Design review of the part built by this model. Coordinates are the model's own, in mm. A direction names the side the tool comes from. Give positions to 0.01 mm unless a question says otherwise; leave off trailing zeros. Loops run counter-clockwise (first coordinate to the right, second up) from the corner with the lowest first, then second, coordinate; pieces in that order, holes last. Notation, with made-up numbers: (-26.5, -32) -> (-6.5, -32) arc R32 ccw to (-6.5, -6) -> close; hole circle Ø5 at (47.5, 77.25). An arc over 180 degrees is marked (long way). Use a Markdown table: item, result. Add a question column.
1. Add section A-A (y = 0). State the section outline as (x, z) points, and give its area (3 significant figures).
2. Add section B-B (z = 22). State the section outline as (x, y) points, and give its area (3 significant figures).
3. Draft analysis for pull direction Y (two halves, no side actions). For faces 1 (the flat face through (-43, 16, 26)), 2 (the flat face through (0, -30, 20)), 3 (the flat face through (9, -35, 3)), 4 (the flat face through (-2, 33, 23)), state which applies: pulls with the +Y half, pulls with the -Y half, needs draft (parallel to the pull), parting line crosses it, or undercut.
4. For faces 5 (the flat face through (-43, 16, 13)), 6 (the flat face through (42, 0, 23)), 7 (the flat face through (-2, 7, 40)), 8 (the flat face through (3.5, 0, 42)), list the 3-axis set-ups (+Z, -Z, +X, -X, +Y, -Y) from which the entire face can be reached by the end or side of a thin tool; tool diameter is ignored.
5. Add section C-C (x = 0). State the section outline as (y, z) points.
6. To check wall thickness, follow line 1 (Y direction, x = 0, z = 0.75); line 2 (X direction, y = -6, z = 34.5); line 3 (Y direction, x = 12.5, z = 11.5). State the ranges of each line that lie inside material, in increasing order.
7. For pin 1 Ø1 at (y, z) = (4.5, 15.5) entering from +X; pin 2 Ø12 at (y, z) = (15, 28.5) entering from -X; pin 3 Ø8 at (x, y) = (0, 40) entering from -Z; pin 4 Ø6 at (y, z) = (-22, 5.5) entering from -X, all flat-tipped, find the tip position at first contact; note any pin that passes through.
8. Add section D-D (z = 35). State the section outline as (x, y) points.
```python
from build123d import *

# Parameters (mm, degrees)
F0_R     = 60
F0_R_2   = 5
F0_W     = 86
F0_H     = 66
F1_DEPTH = 3
F2_DEPTH = 40
F3_W     = 86
F3_H     = 66
F4_DEPTH = 3
F5_W     = 10
F5_H     = 12
F5_W_2   = 13
F5_H_2   = 13
F6_DEPTH = 25
F8_DEPTH = 25


with BuildPart() as f1:
    # F0 (on Top) → F1 (new body)
    with BuildSketch(Plane.XY):
        Circle(F0_R)
        with Locations((0, -40)):
            Circle(F0_R_2, mode=Mode.SUBTRACT)
        with Locations((-1, 0)):
            Rectangle(F0_W, F0_H, mode=Mode.SUBTRACT)
        with Locations((0, 40)):
            Circle(F0_R_2, mode=Mode.SUBTRACT)
    extrude(amount=F1_DEPTH)

    # F0 (on Top) → F2 (join)
    with BuildSketch(Plane.XY):
        with Locations((-1, 0)):
            Rectangle(F0_W, F0_H)
        Polygon((39, 30), (39, 2), (39, -30), (-41, -30), (-41, 0), (-41, 30), align=None, mode=Mode.SUBTRACT)
    extrude(amount=F2_DEPTH)

    # F3 (on face) → F4 (join)
    with BuildSketch(Plane.XY.offset(40)):
        with Locations((-1, 0)):
            Rectangle(F3_W, F3_H)
    extrude(amount=F4_DEPTH)

    # F5 (on face) → F6 (cut)
    with BuildSketch(Plane(origin=(-44, 0, 0), x_dir=(0, -1, 0), z_dir=(-1, 0, 0))):
        with Locations((14.5, 19)):
            Rectangle(F5_W, F5_H)
        with Locations((-15.9, 19.5)):
            Rectangle(F5_W_2, F5_H_2)
    extrude(amount=-F6_DEPTH, mode=Mode.SUBTRACT)

    # F7 (on face) → F8 (cut)
    with BuildSketch(Plane.XY.offset(43)):
        Polygon((3.5, -3.1), (3.5, 0), (3.5, 3.1), (-3.5, 3.1), (-3.5, 0), (-3.5, -3.1), align=None)
    extrude(amount=-F8_DEPTH, mode=Mode.SUBTRACT)


solid = f1.part
```
Taken from the geometry:
| question | item | result |
|---|---|---|
| 1 | outline | (-60, 0) -> (-41, 0) -> (-41, 40) -> (-3.5, 40) -> (-3.5, 43) -> (-44, 43) -> (-44, 3) -> (-60, 3) -> close; (3.5, 40) -> (39, 40) -> (39, 0) -> (60, 0) -> (60, 3) -> (42, 3) -> (42, 43) -> (3.5, 43) -> close |
| 1 | area | 579 mm^2 |
| 2 | outline | (-44, -33) -> (42, -33) -> (42, 33) -> (-44, 33) -> (-44, 22.4) -> (-41, 22.4) -> (-41, 30) -> (39, 30) -> (39, -30) -> (-41, -30) -> (-41, -19.5) -> (-44, -19.5) -> close; (-44, -9.5) -> (-41, -9.5) -> (-41, 9.4) -> (-44, 9.4) -> close |
| 2 | area | 807 mm^2 |
| 3 | face 1 | undercut |
| 3 | face 2 | undercut |
| 3 | face 3 | needs draft |
| 3 | face 4 | pulls with the +Y half |
| 4 | face 5 | -X |
| 4 | face 6 | +Z, +X, +Y, -Y |
| 4 | face 7 | -Z |
| 4 | face 8 | +Z, -Z |
| 5 | outline | (-60, 0) -> (-45, 0) -> (-45, 3) -> (-60, 3) -> close; (-35, 0) -> (-30, 0) -> (-30, 40) -> (-3.1, 40) -> (-3.1, 43) -> (-33, 43) -> (-33, 3) -> (-35, 3) -> close; (3.1, 40) -> (30, 40) -> (30, 0) -> (35, 0) -> (35, 3) -> (33, 3) -> (33, 43) -> (3.1, 43) -> close; (45, 0) -> (60, 0) -> (60, 3) -> (45, 3) -> close |
| 6 | line 1 | y = -60 to -45, -35 to -30, 30 to 35, 45 to 60 |
| 6 | line 2 | x = -44 to -41, 39 to 42 |
| 6 | line 3 | y = -33 to -30, 30 to 33 |
| 7 | pin 1 | stops at x = 42 |
| 7 | pin 2 | stops at x = -44 |
| 7 | pin 3 | passes through |
| 7 | pin 4 | stops at x = -56.45 |
| 8 | outline | (-44, -33) -> (42, -33) -> (42, 33) -> (-44, 33) -> close; hole (-41, -30) -> (39, -30) -> (39, 30) -> (-41, 30) -> close |
